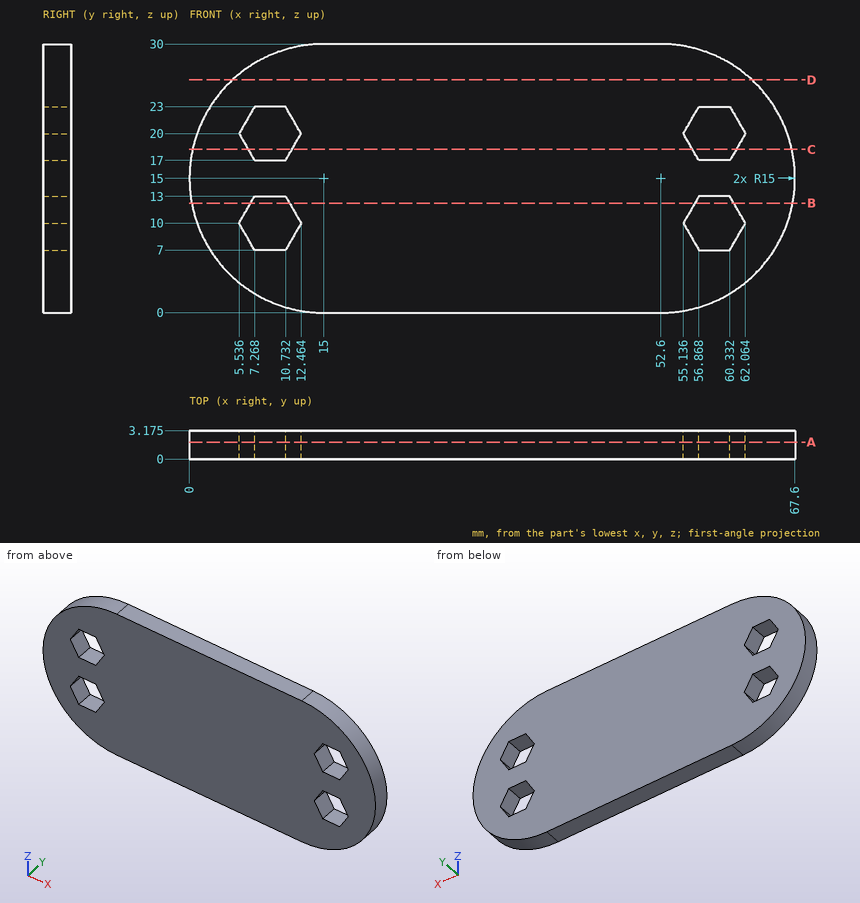
Study the drawing (mm; zero at the part's minimum x, y, z) and answer. Round coordinates to 2 decimals unless told otherwise and drop trailing zeros. Write each loop counter-clockwise with the first axis right and the second up, starting at its lowest first coordinate (ties: lowest second). Pieces come first, ordered by that corner, then holes. Notation, with made-up numbers: (-16.75, 27) - (31.25, 27) arc R28 ccw to (31.25, 58) - close; hole circle Ø2 at (25.25, 75). An arc over 180 degrees is marked (long way). Use a Markdown table: item, result. Add a question column.
1. Flat-ended cylindrical pins translate along their axes: P1, Ø1, axis at x = 59, y = 1, coming from the +Z side; P2, Ø1, axis at x = 59.5, y = 1.5, coming from the -Z side; P3, Ø1.6, axis at x = 9, y = 1.5, coming from the -Z side; P4, Ø12, axis at x = 48.5, z = 25, coming from the -Y side. Find the tip coordinate at first contact, or state that the pin passes through.
2. The part is cut by section A-A (y = 1.9). Write down the section's boundary in (x, z).
3. The part is cut by section D-D (z = 26). Write down the section's boundary in (x, y) (3 decimals).
4. The part is cut by section B-B (z = 12.25). Write down the section's boundary in (x, y) (3 decimals), and give its area (4 significant figures).
5. Consider line 1 (X direction, y = 1.9, z = 22); line 2 (X direction, y = 1.4, z = 15); line 3 (X direction, y = 0.7, z = 10.5) (1 decimal). Determine where each line is inside the solid, lowest interval first.
6. The part is cut by section C-C (z = 18.25). Write down the section's boundary in (x, y) (1 decimal).
Reported:
| question | item | result |
|---|---|---|
| 1 | P1 | z = 28.79 |
| 1 | P2 | z = 1.43 |
| 1 | P3 | z = 0.93 |
| 1 | P4 | y = 0 |
| 2 | outline | (15, 0) - (52.6, 0) arc R15 ccw to (52.6, 30) - (15, 30) arc R15 ccw to start; hole (5.54, 10) - (7.27, 7) - (10.73, 7) - (12.46, 10) - (10.73, 13) - (7.27, 13) - close; hole (5.54, 20) - (7.27, 17) - (10.73, 17) - (12.46, 20) - (10.73, 23) - (7.27, 23) - close; hole (55.14, 10) - (56.87, 7) - (60.33, 7) - (62.06, 10) - (60.33, 13) - (56.87, 13) - close; hole (55.14, 20) - (56.87, 17) - (60.33, 17) - (62.06, 20) - (60.33, 23) - (56.87, 23) - close |
| 3 | outline | (4.802, 0) - (62.798, 0) - (62.798, 3.175) - (4.802, 3.175) - close |
| 4 | outline | (0.254, 0) - (6.835, 0) - (6.835, 3.175) - (0.254, 3.175) - close; (11.165, 0) - (56.435, 0) - (56.435, 3.175) - (11.165, 3.175) - close; (60.765, 0) - (67.346, 0) - (67.346, 3.175) - (60.765, 3.175) - close |
| 4 | area | 185.5 mm^2 |
| 5 | line 1 | 1.73 to 6.69, 11.31 to 56.29, 60.91 to 65.87 |
| 5 | line 2 | 0 to 67.6 |
| 5 | line 3 | 0.7 to 5.8, 12.2 to 55.4, 61.8 to 66.9 |
| 6 | outline | (0.4, 0) - (6.5, 0) - (6.5, 3.2) - (0.4, 3.2) - close; (11.5, 0) - (56.1, 0) - (56.1, 3.2) - (11.5, 3.2) - close; (61.1, 0) - (67.2, 0) - (67.2, 3.2) - (61.1, 3.2) - close |
